```python
from build123d import *

# Parameters (mm, degrees)
PAD_DEPTH    = 14
PAD001_DEPTH = 13
POCKET_DEPTH = 100
SKETCH003_W  = 4.75
SKETCH003_H  = 5
PAD002_DEPTH = 14
FILLET_R     = 1
FILLET001_R  = 1


with BuildPart() as part:
    # Sketch → Pad (new body)
    with BuildSketch(Plane.YZ):
        Polygon((0, 0), (0, 15), (2, 15), (2, 2), (54, 2), (54, 42), (56, 42), (56, 0), align=None)
    extrude(amount=PAD_DEPTH)

    # Sketch001 (on Face4 of Pad) → Pad001 (join)
    with BuildSketch(Plane(origin=(0, 0, 2), x_dir=(0, -1, 0), z_dir=(0, 0, 1))):
        with BuildLine():
            Line((-2, 14), (-2.987861, 14))
            ThreePointArc((-4.342771, 0), (-3.593472, 6.993047), (-2.987861, 14))
            Line((-2, 0), (-4.342771, 0))
            Line((-2, 0), (-2, 14))
        make_face()
    extrude(amount=PAD001_DEPTH)

    # Sketch002 (on Face10 of Pad001) → Pocket (cut)
    with BuildSketch(Plane.YZ.offset(14)):
        with BuildLine():
            ThreePointArc((2.987861, 15), (4.153127, 9.106971), (5.487861, 3.25))
            Line((5.487861, 15), (5.487861, 3.25))
            Line((2.987861, 15), (5.487861, 15))
        make_face()
    extrude(amount=-POCKET_DEPTH, mode=Mode.SUBTRACT)

    # Sketch003 (on Face2 of Pocket) → Pad002 (join)
    with BuildSketch(Plane(origin=(0, 0, 0), x_dir=(0, 1, 0), z_dir=(-1, 0, 0))):
        with Locations((51.625, -4.5)):
            Rectangle(SKETCH003_W, SKETCH003_H)
    extrude(amount=-PAD002_DEPTH)

    # Fillet
    fillet_edges = [part.edges().sort_by_distance(p)[0] for p in [
        (7, 49.25, 7),
    ]]
    fillet(fillet_edges, radius=FILLET_R)

    # Fillet001
    fillet001_edges = [part.edges().sort_by_distance(p)[0] for p in [
        (7, 54, 7),
    ]]
    fillet(fillet001_edges, radius=FILLET001_R)


solid = part.part
```
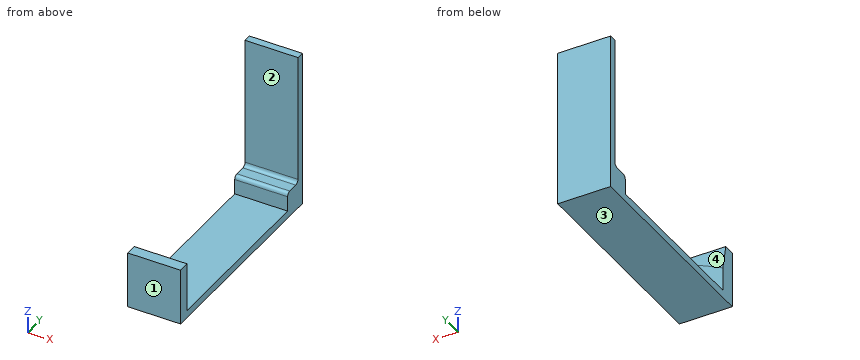
The model under review builds one solid part; all positions refer to its coordinate system, in mm. Face numbers are marked on the shaded views. Round coordinates to 2 decimals unless told otherwise and drop trailing zeros. Loops run counter-clockwise (first coordinate to the right, second up) from the corner with the lowest first, then second, coordinate; pieces in that order, holes last. Notation, with made-up numbers: M 84,1.5 L 88,1.5 A22 ccw 88,28.5 Z; hole C 2.5,76.25 d4. An arc over 180 degrees is marked long. Write item = value, one per line.
Item 1: Take a section at C-C on y = 28.5. Write out the cut boundary in (x, z), then the cut area to 3 significant figures.
Return value:
outline = M 0,0 L 14,0 L 14,2 L 0,2 Z
area = 28.0 mm2
Item 2: For line 1 (Z direction, x = 7.75, y = 9); line 2 (Y direction, x = 2.75, z = 19); line 3 (Y direction, x = 11.5, z = 12), list the stretches that pass through material, from the lowest coordinate up. Write a range as [from, to].
Return value:
line_1 = [0, 2]
line_2 = [54, 56]
line_3 = [0, 3.19], [54, 56]
Item 3: Take a section at A-A on z = 9. Write out the cut boundary in (x, y), then the cut area to 3 significant figures.
Return value:
outline = M 0,0 L 14,0 L 14,2.99 A342.65 cw 1.45,4.18 L 0,4.18 Z; M 0,54 L 14,54 L 14,56 L 0,56 Z
area = 78.5 mm2
Item 4: The part is to be moulded in two halves that separate along Y. For the marked faces 1, 2, 3 and 4, say which applies: released by +Y, released by -Y, zero draft, split by the parting line, or undercut.
Return value:
face_1 = released by -Y
face_2 = undercut
face_3 = zero draft
face_4 = undercut
Item 5: Take a section at B-B on x = 12.5. Write out the cut boundary in (y, z).
Return value:
outline = M 0,0 L 56,0 L 56,42 L 54,42 L 54,8 A1 cw 53,7 L 50.25,7 A1 ccw 49.25,6 L 49.25,2 L 3.11,2 L 3.11,14.36 A208.27 cw 2.99,15 L 0,15 Z
Item 6: Take a section at D-D on x = 3. Write out the cut boundary in (y, z), then the cut area to 3 significant figures.
Return value:
outline = M 0,0 L 56,0 L 56,42 L 54,42 L 54,8 A1 cw 53,7 L 50.25,7 A1 ccw 49.25,6 L 49.25,2 L 4,2 L 4,9.82 A208.27 cw 2.99,15 L 0,15 Z
area = 265 mm2
Item 7: Insertion check: P1, Ø1.5, axis at x = 8.5, y = 9.5, coming from the +Z side; P2, Ø1.4, axis at x = 10.5, y = 51.5, coming from the +Z side; P3, Ø3.5, axis at x = 8, y = 1.5, coming from the +Z side. Each pin has a flat end and moves straight along its axis. Give the tip position at first contact, or say it passes through.
Return value:
P1 = 2
P2 = 7
P3 = 15
